For this review, take the finished solid that the model builds, in its own axes (mm). A direction names the side the tool comes from. Give positions to 0.01 mm unless a question says otherwise; leave off trailing zeros. Loops run counter-clockwise (first coordinate to the right, second up) from the corner with the lowest first, then second, coordinate; pieces in that order, holes last. Notation, with made-up numbers: (75.5, 28.5) - (97.5, 28.5) arc R31 ccw to (97.5, 67.5) - close; hole circle Ø8 at (3.5, -3). An arc over 180 degrees is marked (long way). Put each result on its own line as item: value.
from build123d import *

# Parameters (mm, degrees)
SM_BASE_FLANGE_1_DEPTH = 135
SKETCH_2_R             = 2.5
CUT_EXTRUDE_1_DEPTH    = 10


# Sheet-metal steps are written as plain solids
with BuildPart() as part:
    # Sketch 1 → Базовая кромка1 (new, symmetric)
    with BuildSketch(Plane.XY):
        with BuildLine():
            Line((-13.5, -10.5), (-13.5, -1.5))
            ThreePointArc((-13.5, -1.5), (-13.060660172, -0.439339828), (-12, 0))
            Line((-12, 0), (12, 0))
            ThreePointArc((12, 0), (13.060660172, -0.439339828), (13.5, -1.5))
            Line((13.5, -1.5), (13.5, -10.5))
            Line((13.5, -10.5), (15, -10.5))
            Line((15, -10.5), (15, -1.5))
            ThreePointArc((15, -1.5), (14.121320344, 0.621320344), (12, 1.5))
            Line((12, 1.5), (-12, 1.5))
            ThreePointArc((-12, 1.5), (-14.121320344, 0.621320344), (-15, -1.5))
            Line((-15, -1.5), (-15, -10.5))
            Line((-15, -10.5), (-13.5, -10.5))
        make_face()
    extrude(amount=SM_BASE_FLANGE_1_DEPTH, both=True)

    # Sketch 2 → Вырез-Вытянуть1 (cut)
    with BuildSketch(Plane(origin=(0, 1.5, 0), x_dir=(1, 0, 0), z_dir=(0, 1, 0))):
        with Locations(Location((0, 0, 0), (0, 0, 180))):
            Circle(SKETCH_2_R)
        with Locations((0, 460)):
            Circle(SKETCH_2_R)
        with Locations(Location((0, -115, 0), (0, 0, 180))):
            Circle(SKETCH_2_R)
        with Locations((0, -230)):
            Circle(SKETCH_2_R)
        with Locations((0, -345)):
            Circle(SKETCH_2_R)
        with Locations((0, -460)):
            Circle(SKETCH_2_R)
        with Locations(Location((0, 115, 0), (0, 0, 180))):
            Circle(SKETCH_2_R)
        with Locations((0, 230)):
            Circle(SKETCH_2_R)
        with Locations((0, 345)):
            Circle(SKETCH_2_R)
    extrude(amount=-CUT_EXTRUDE_1_DEPTH, mode=Mode.SUBTRACT)


solid = part.part
1) Take a section at A-A on y = -4.75. State the section outline as (x, z) points, and give its area (3 significant figures).
Geometry check:
outline: (-15, -135) - (-13.5, -135) - (-13.5, 135) - (-15, 135) - close; (13.5, -135) - (15, -135) - (15, 135) - (13.5, 135) - close
area: 810 mm²
2) Take a section at D-D on x = 6.5. State the section outline as (y, z) points, and give its area (3 significant figures).
Geometry check:
outline: (0, -135) - (1.5, -135) - (1.5, 135) - (0, 135) - close
area: 405 mm²
3) Insertion check: pin 1 Ø1 at (y, z) = (-0.5, 51) entering from -X; pin 2 Ø6.5 at (x, z) = (0, -115) entering from -Y; pin 3 Ø3 at (x, z) = (0, 0) entering from +Y. Each pin has a flat end and moves straight along its axis. Give the tip position at first contact, or say it passes through.
Geometry check:
pin 1: stops at x = -14.96
pin 2: stops at y = 0
pin 3: passes through
4) Take a section at C-C on z = 101. State the section outline as (x, y) points, and give its area (3 significant figures).
Geometry check:
outline: (-15, -10.5) - (-13.5, -10.5) - (-13.5, -1.5) arc R1.5 cw to (-12, 0) - (12, 0) arc R1.5 cw to (13.5, -1.5) - (13.5, -10.5) - (15, -10.5) - (15, -1.5) arc R3 ccw to (12, 1.5) - (-12, 1.5) arc R3 ccw to (-15, -1.5) - close
area: 73.6 mm²
5) For faces 1 (the face through (-2, 1.5, 2)), 2 (the face through (13.5, -6, 2)), list the 3-axis set-ups (+Z, -Z, +X, -X, +Y, -Y) from which the entire face can be reached by the end or side of a thin tool; tool diameter is ignored.
Geometry check:
face 1: +Z, -Z, +X, -X, +Y
face 2: +Z, -Z, -Y
6) Draft analysis for pull direction X (two halves, no side actions). For faces 3 (the face through (-0.1, 0.4, -135)), 4 (the face through (2, 0, 2)), 5 (the face through (-13.5, -6, 2)), 6 (the face through (-15, -6, 2)), state which applies: pulls with the +X half, pulls with the -X half, needs draft (parallel to the pull), parting line crosses it, or undercut.
Geometry check:
face 3: needs draft
face 4: undercut
face 5: undercut
face 6: pulls with the -X half
7) Wall thickness on line 1 (Z direction, x = 0, y = 0.6); line 2 (X direction, y = -5.75, z = -76); line 3 (Y direction, x = 10.25, z = -97.5): over which ranges is each line inside the solid? List them lowest first.
Geometry check:
line 1: z = -135 to -117.5, -112.5 to -2.5, 2.5 to 112.5, 117.5 to 135
line 2: x = -15 to -13.5, 13.5 to 15
line 3: y = 0 to 1.5
8) Take a section at B-B on z = -115. State the section outline as (x, y) points.
Geometry check:
outline: (-15, -10.5) - (-13.5, -10.5) - (-13.5, -1.5) arc R1.5 cw to (-12, 0) - (-2.5, 0) - (-2.5, 1.5) - (-12, 1.5) arc R3 ccw to (-15, -1.5) - close; (2.5, 0) - (12, 0) arc R1.5 cw to (13.5, -1.5) - (13.5, -10.5) - (15, -10.5) - (15, -1.5) arc R3 ccw to (12, 1.5) - (2.5, 1.5) - close
